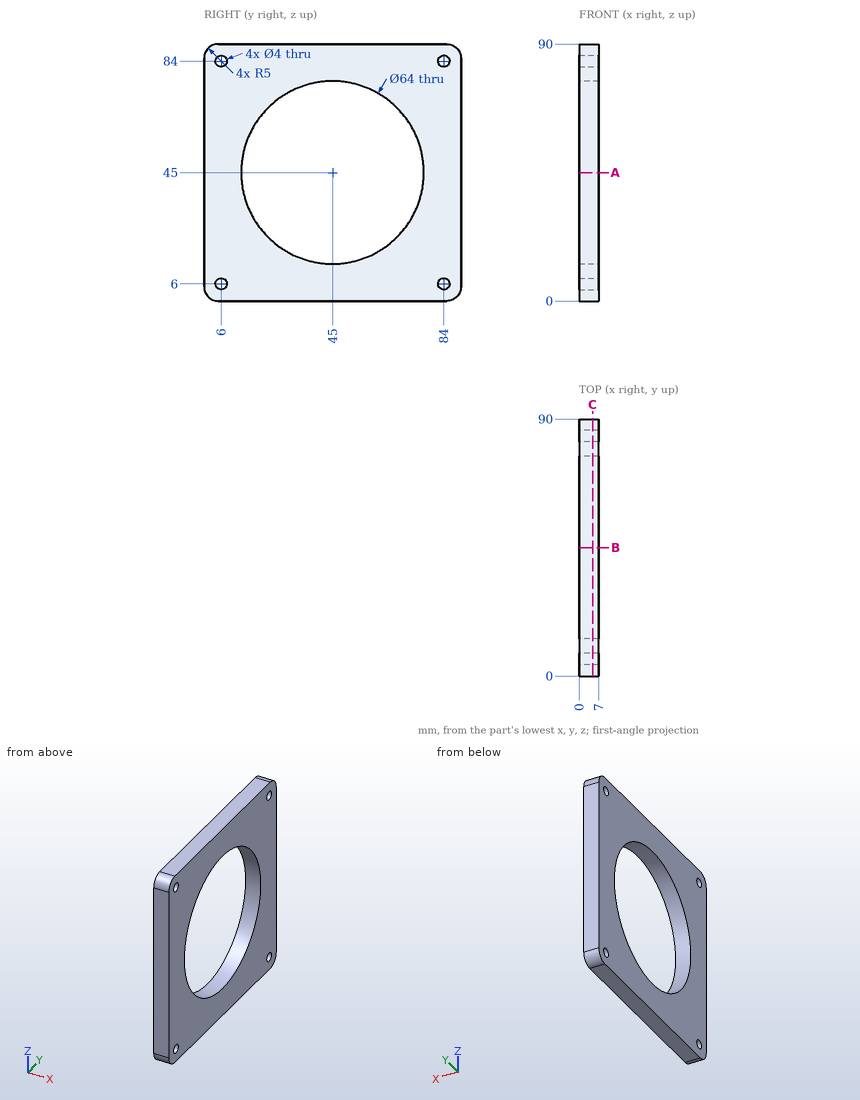
For this review, use the dimensioned drawing (mm, ordinates from the lowest corner) and the shaded views. Round coordinates to 2 decimals unless told otherwise and drop trailing zeros. Write each loop counter-clockwise with the first axis right and the second up, starting at its lowest first coordinate (ties: lowest second). Pieces come first, ordered by that corner, then holes. Notation, with made-up numbers: (47.25, 57.25) - (94.25, 57.25) arc R23 cw to (94.25, 66.25) - close; hole circle Ø3 at (60, 26). An arc over 180 degrees is marked (long way). One line per item, written item: value. Start each with the question number.
1. To check wall thickness, follow L1, parallel to Z at x = 3, y = 84; L2, parallel to Z at x = 1.5, y = 83. State the ranges of each line that lie inside material, in increasing order. Write a range as from..to.
2. Consider section A-A on z = 45. Write out the cut boundary in (x, y), and give its area (3 significant figures).
3. Clearance check with a flat-ended pin moving along its axis: P1, Ø4.5, axis at y = 6, z = 6, coming from the -X side. State where the tip first meets the part, or that it passes through.
4. Consider section C-C on x = 4.75. Write out the cut boundary in (y, z).
Checks:
1. L1: z = 0..4, 8..82, 86..90
1. L2: z = 0..4.27, 7.73..82.27, 85.73..90
2. outline: (0, 0) - (7, 0) - (7, 13) - (0, 13) - close; (0, 77) - (7, 77) - (7, 90) - (0, 90) - close
2. area: 182 mm^2
3. P1: stops at x = 0
4. outline: (0, 5) arc R5 ccw to (5, 0) - (85, 0) arc R5 ccw to (90, 5) - (90, 85) arc R5 ccw to (85, 90) - (5, 90) arc R5 ccw to (0, 85) - close; hole circle Ø4 at (6, 6); hole circle Ø4 at (6, 84); hole circle Ø64 at (45, 45); hole circle Ø4 at (84, 6); hole circle Ø4 at (84, 84)
